from build123d import *

# Parameters (mm, degrees)
F3_DEPTH      = 177.8
F3_DEPTH_BACK = 12.7
F4_R          = 7.62
F5_DEPTH      = 19.05
F6_SIZE2      = 18.860161823
F6_SIZE       = 7.62
F4_R_2        = 5.715
F7_DEPTH      = 5.08
F8_R          = 5.07999
F9_R          = 6.139399456
F10_DEPTH     = 50.8
F11_SCALE     = 0.51715159


# Not quite as in the source:
# - a fillet or chamfer is up to 0.001 mm smaller than in the source, because OpenCascade refuses the exact size


with BuildPart() as f1:
    # F0 (on Front) → F1 (revolve)
    with BuildSketch(Plane.XZ):
        with BuildLine():
            Line((-6.139399456, 0), (0, 0))
            Line((0, 0), (0, 146.0500033258))
            Line((0, 146.0500033258), (0, 152.4))
            ThreePointArc((0, 152.4), (-33.2006597867, 137.6319951518), (-44.4655865431, 103.0852268133))
            add(Edge.make_bspline(
                [(-49.1152013464, 36.1084283333), (-48.0326439436, 49.6014705241), (-37.8272166921, 76.0482431769), (-42.543614325, 94.8604386904), (-44.4655865431, 103.0852268133)],
                knots=[0.3424224234, 0.3424224234, 0.3424224234, 0.3424224234, 0.7066775859, 1, 1, 1, 1], degree=3))
            Line((-49.1152013464, 36.1084283333), (-49.1152013464, 25.6455829718))
            add(Edge.make_bspline(
                [(-44.4655865431, 0), (-46.3688797408, 8.4610342592), (-48.4665187415, 16.8703142107), (-49.1152013464, 25.6455829718)],
                knots=[0, 0, 0, 0, 0.246321171, 0.246321171, 0.246321171, 0.246321171], degree=3))
            Line((-44.4655865431, 0), (-38.2711647941, 0))
            Line((-38.2711647941, 0), (-6.139399456, 0))
        make_face()
        Polygon((-6.139399456, -6.35), (-6.139399456, 0), (-38.2711647941, 0), (-44.4655865431, 0), (-44.4655865431, -6.35), align=None)
        with BuildLine():
            Line((-44.4655865431, -6.35), (-44.4655865431, 0))
            add(Edge.make_bspline(
                [(-44.4655865431, 0), (-46.3688797408, 8.4610342592), (-48.4665187415, 16.8703142107), (-49.1152013464, 25.6455829718)],
                knots=[0, 0, 0, 0, 0.246321171, 0.246321171, 0.246321171, 0.246321171], degree=3))
            Line((-49.1152013464, 25.6455829718), (-49.1152013464, 0))
            Line((-49.1152013464, 0), (-49.1152013464, -6.35))
            Line((-49.1152013464, -6.35), (-44.4655865431, -6.35))
        make_face()
        with BuildLine():
            add(Edge.make_bspline(
                [(-49.1152013464, 25.6455829718), (-49.3682823563, 29.0692201465), (-49.4008119098, 32.5485659437), (-49.1152013464, 36.1084283333)],
                knots=[0.246321171, 0.246321171, 0.246321171, 0.246321171, 0.3424224234, 0.3424224234, 0.3424224234, 0.3424224234], degree=3))
            Line((-49.1152013464, 25.6455829718), (-49.1152013464, 36.1084283333))
        make_face()
    revolve(axis=Axis((0, 0, 76.2), (0, 0, 1)))

    # F2 (on Top) → F3 (cut, two sides)
    with BuildSketch(Plane.XY) as f3_sk:
        Polygon((25.6092443837, -36.641700535), (-25.1907556163, -36.641700535), (-46.7807556163, -36.641700535), (-46.7807556163, -67.121700535), (42.1192443837, -67.121700535), (42.1192443837, -36.641700535), align=None)
    extrude(amount=F3_DEPTH, mode=Mode.SUBTRACT)
    extrude(f3_sk.sketch, amount=-F3_DEPTH_BACK, mode=Mode.SUBTRACT)

    # F4 (on face) → F5 (join)
    with BuildSketch(Plane.XZ.offset(36.641700535)):
        with Locations((0, 97.9992443837)):
            Circle(F4_R)
    extrude(amount=F5_DEPTH)

    # F6
    f6_edges = [f1.edges().sort_by_distance(p)[0] for p in [
        (-7.62, -55.691701, 97.999244),
    ]]
    f6_side = f1.faces().sort_by_distance((0, -55.691701, 97.999244))[0]
    chamfer(f6_edges, length=F6_SIZE, length2=F6_SIZE2, reference=f6_side)

    # F4 (on face) → F7 (join)
    with BuildSketch(Plane.XZ.offset(36.641700535)):
        with Locations((-12.7, 112.2232443837)):
            Circle(F4_R_2)
        with Locations((12.7, 112.2232443837)):
            Circle(F4_R_2)
    extrude(amount=F7_DEPTH)

    # F8 (radius 5.08 in the source; OpenCascade refuses exactly that, so slightly less here)
    f8_edges = [f1.edges().sort_by_distance(p)[0] for p in [
        (-18.415, -41.721701, 112.223244),
        (6.985, -41.721701, 112.223244),
    ]]
    fillet(f8_edges, radius=F8_R)

    # F9 (on face) → F10 (cut)
    with BuildSketch(Plane(origin=(0, 0, -6.35), x_dir=(1, 0, 0), z_dir=(0, 0, -1))):
        Circle(F9_R)
    extrude(amount=-F10_DEPTH, mode=Mode.SUBTRACT)


with BuildPart() as f1_1:
    # F11: moved
    add(f1.part.scale(F11_SCALE))


solid = f1_1.part
Model file for the job. Use its own axes, mm. Round coordinates to 2 decimals unless told otherwise and drop trailing zeros.
1. Wall check: probe 1 along X at (y, z) = (0, 10) (3 decimals); probe 2 along Y at (x, z) = (0, 7) (3 decimals); probe 3 along Y at (x, z) = (-7, 26). Give the ranges that are in metal, low to high.
Check values:
probe 1: x = -25.4 to -3.175, 3.175 to 25.4
probe 2: y = -18.949 to -3.175, 3.175 to 25.4
probe 3: y = -18.95 to 23.14
2. Mould opens along X. For faces 1 (the conical face through (0.839, -24.94, 51.996)), 2 (the flat face through (0, 0, 22.987)), 3 (the flat face through (-5, 3, -3.284)) say: +X half, -X half, draft (parallel to the pull), parting line (faces both ways), or undercut.
Check values:
face 1: parting line
face 2: undercut
face 3: draft
3. Drop flat-ended pins along their axis: P1, Ø1, axis at y = -12, z = 69.5, coming from the +X side; P2, Ø10, axis at y = -3.5, z = 57, coming from the +X side; P3, Ø10, axis at x = 8, z = 33, coming from the -Y side; P4, Ø7, axis at x = -0.5, y = 0.5, coming from the -Z side. Give the stop position or say it passes through.
Check values:
P1: stops at x = 14.76
P2: stops at x = 23.12
P3: stops at y = -18.95
P4: stops at z = -3.28
